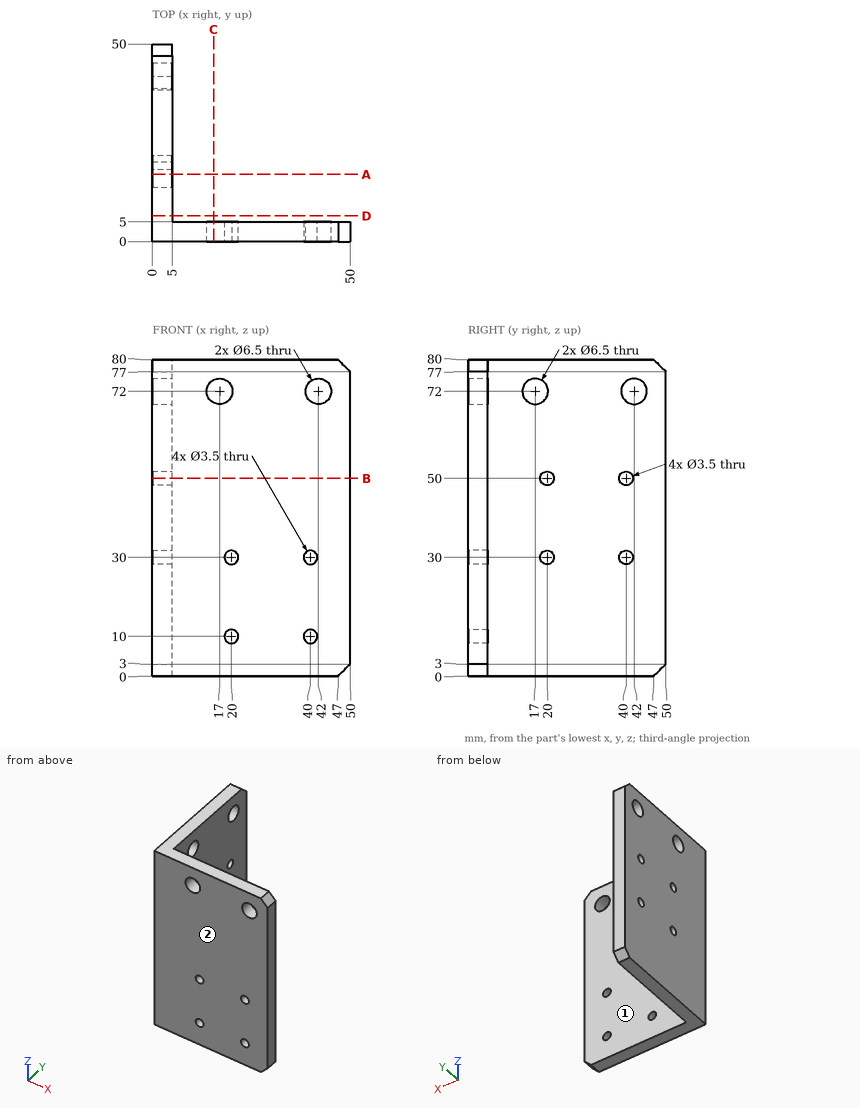
Source: three-view drawing plus pictorial views. Frame: mm from the lowest corner of the part. A direction names the side the tool comes from. Round coordinates to 2 decimals unless told otherwise and drop trailing zeros. Loops run counter-clockwise (first coordinate to the right, second up) from the corner with the lowest first, then second, coordinate; pieces in that order, holes last. Notation, with made-up numbers: M 50.5,-25.5 L 64.5,-25.5 A17 cw 64.5,-15.5 Z; hole C 77.5,81.25 d10. An arc over 180 degrees is marked long. Answer as CSV lines item,"result".
Q1. Cut plane D-D (y = 6.5). Return the cut outline in (x, z).
Verdict:
outline,"M 0,0 L 5,0 L 5,80 L 0,80 Z"
Q2. Cut plane C-C (x = 15.5). Return the cut outline in (y, z), plus the area to 3 significant figures.
Verdict:
outline,"M 0,0 L 5,0 L 5,69.12 L 0,69.12 Z; M 0,74.88 L 5,74.88 L 5,80 L 0,80 Z"
area,"371 mm^2"
Q3. Line query: line 1 along Y through (x, z) = (3.9, 30); line 2 along Y through (x, z) = (3.6, 72); line 3 along Z through (x, y) = (20, 2.55). Output: solid intervals per line, ascending.
Verdict:
line 1,"y = 0 to 18.25, 21.75 to 38.25, 41.75 to 50"
line 2,"y = 0 to 13.75, 20.25 to 38.75, 45.25 to 50"
line 3,"z = 0 to 8.25, 11.75 to 28.25, 31.75 to 70.75, 73.25 to 80"
Q4. Cut plane A-A (y = 17). Return the cut outline in (x, z).
Verdict:
outline,"M 0,0 L 5,0 L 5,68.75 L 0,68.75 Z; M 0,75.25 L 5,75.25 L 5,80 L 0,80 Z"
Q5. Cut plane B-B (z = 50). Return the cut outline in (x, y), plus the area to 3 significant figures.
Verdict:
outline,"M 0,0 L 50,0 L 50,5 L 5,5 L 5,18.25 L 0,18.25 Z; M 0,21.75 L 5,21.75 L 5,38.25 L 0,38.25 Z; M 0,41.75 L 5,41.75 L 5,50 L 0,50 Z"
area,"440 mm^2"
Q6. Reachability of the marked faces 1 and 2 from +Z, -Z, +X, -X, +Y, -Y: full face, straight path, thin tool, end or side. Return the list, or none.
Verdict:
face 1,"+Z, -Z, +X, +Y"
face 2,"+Z, -Z, +X, -X, -Y"
Q7. Contact query for flat-ended pins moving along their axis: pin 1 (4.5 mm diameter, centred on x = 20, z = 10, fed in from +Y); pin 2 (4 mm diameter, centred on y = 17, z = 72, fed in from -X); pin 3 (4.5 mm diameter, centred on y = 20, z = 50, fed in from +X). Output: stop coordinate, or through.
Verdict:
pin 1,"stops at y = 5"
pin 2,"passes through"
pin 3,"stops at x = 5"
